The listing builds one solid part. Answer for the finished solid, in the listing's coordinates (mm). A direction names the side the tool comes from. Round coordinates to 2 decimals unless told otherwise and drop trailing zeros. Order: outer loops, then holes, each group sorted by start corner. A loop starts at its lowest first (then second) coordinate and runs counter-clockwise, first axis right, second up. Notation, with made-up numbers: (-18, 43) - (-1, 43) arc R25 ccw to (-1, 79) - close; hole circle Ø8 at (81.5, 70.25). An arc over 180 degrees is marked (long way). Write item = value, one per line.
from build123d import *

# Parameters (mm, degrees)
SKETCH1_W            = 20
SKETCH1_H            = 20
BOSS_EXTRUDE1_DEPTH  = 7.5
SKETCH1_3_W          = 20
SKETCH1_3_H          = 20
CUT_EXTRUDE2_DEPTH   = 1.5
SKETCH3_W            = 10
SKETCH3_H            = 20
BOSS_EXTRUDE2_DEPTH  = 1.5
SKETCH4_R            = 1.5
CUT_EXTRUDE3_DEPTH   = 5
MOUNTHOLE_DEPTH      = 17.007810594
MOUNTHOLE_DEPTH_BACK = 17.007810594
SKETCH5_R            = 1.5
SKETCH6_R            = 3
CUT_EXTRUDE5_DEPTH   = 1.25


with BuildPart() as part:
    # Sketch1 → Boss-Extrude1 (new, symmetric)
    with BuildSketch(Plane(origin=(0, 0, 0), x_dir=(1, 0, 0), z_dir=(0, 1, 0))):
        Rectangle(SKETCH1_W, SKETCH1_H)
    extrude(amount=BOSS_EXTRUDE1_DEPTH, both=True)

    # Sketch1_3 → Cut-Extrude2 (cut, symmetric)
    with BuildSketch(Plane(origin=(0, 0, 0), x_dir=(1, 0, 0), z_dir=(0, 1, 0))):
        Rectangle(SKETCH1_3_W, SKETCH1_3_H)
    extrude(amount=CUT_EXTRUDE2_DEPTH, both=True, mode=Mode.SUBTRACT)


with BuildPart() as cut_extrude2_piece_1:
    # of the separate pieces the step leaves, piece 1, a body of its own (cut_extrude2_pieces)
    add(part.part.solids().sort_by_distance((-10, -7.5, -10))[0])



with BuildPart() as cut_extrude2_piece_2:
    # of the separate pieces the step leaves, piece 2, a body of its own (cut_extrude2_pieces)
    add(part.part.solids().sort_by_distance((-10, 1.5, -10))[0])


with BuildPart() as cut_extrude2_piece_1_1:
    add(cut_extrude2_piece_1.part)

    add(cut_extrude2_piece_2.part)  # Boss-Extrude2 merges Cut-Extrude2 piece 2
    # Sketch3 → Boss-Extrude2 (add, symmetric)
    with BuildSketch(Plane(origin=(0, 0, 0), x_dir=(1, 0, 0), z_dir=(0, 1, 0))):
        with Locations((5, 0)):
            Rectangle(SKETCH3_W, SKETCH3_H)
    extrude(amount=BOSS_EXTRUDE2_DEPTH, both=True)

    # Sketch4 → Cut-Extrude3 (cut)
    with BuildSketch(Plane(origin=(10, 0, 0), x_dir=(0, 0, -1), z_dir=(1, 0, 0))):
        Circle(SKETCH4_R)
    extrude(amount=-CUT_EXTRUDE3_DEPTH, mode=Mode.SUBTRACT)

    # Sketch5 → mounthole (cut, two sides: drawn at the far end of the back side and taken through both)
    with BuildSketch(Plane(origin=(0, 0, 0), x_dir=(1, 0, 0), z_dir=(0, 1, 0)).offset(-MOUNTHOLE_DEPTH_BACK)):
        with Locations(Location((-5, 5, 0), (0, 0, 270))):
            Circle(SKETCH5_R)
        with Locations(Location((5, 5, 0), (0, 0, 270))):
            Circle(SKETCH5_R)
        with Locations(Location((5, -5, 0), (0, 0, 270))):
            Circle(SKETCH5_R)
        with Locations(Location((-5, -5, 0), (0, 0, 270))):
            Circle(SKETCH5_R)
    extrude(amount=MOUNTHOLE_DEPTH + MOUNTHOLE_DEPTH_BACK, mode=Mode.SUBTRACT)

    # Sketch6 → Cut-Extrude5 (cut, symmetric)
    with BuildSketch(Plane(origin=(5, 0, 0), x_dir=(0, 0, -1), z_dir=(1, 0, 0))):
        Circle(SKETCH6_R)
    extrude(amount=CUT_EXTRUDE5_DEPTH, both=True, mode=Mode.SUBTRACT)


solid = cut_extrude2_piece_1_1.part
Q1. Determine the mould class of faces 4 (the face through (-5, 1.5, 0)), 5 (the face through (-3.99, -4.54, -6.11)), 6 (the face through (0, -7.5, 0)) for opening direction Y: released by +Y, released by -Y, zero draft, split by the parting line, or undercut.
Model answer:
face_4 = undercut
face_5 = zero draft
face_6 = released by -Y
Q2. Section A-A on x = -2.75 is taken. Determine the outline of the cut face in (y, z).
Model answer:
outline = (-7.5, -10) - (-1.5, -10) - (-1.5, 10) - (-7.5, 10) - close; (1.5, -10) - (7.5, -10) - (7.5, 10) - (1.5, 10) - close
Q3. Section D-D on z = 5 is taken. Determine the outline of the cut face in (x, y), then the cut area to 3 significant figures.
Model answer:
outline = (-10, -7.5) - (-6.5, -7.5) - (-6.5, -1.5) - (-10, -1.5) - close; (-10, 1.5) - (-6.5, 1.5) - (-6.5, 7.5) - (-10, 7.5) - close; (-3.5, -7.5) - (3.5, -7.5) - (3.5, 7.5) - (-3.5, 7.5) - (-3.5, 1.5) - (0, 1.5) - (0, -1.5) - (-3.5, -1.5) - close; (6.5, -7.5) - (10, -7.5) - (10, 7.5) - (6.5, 7.5) - close
area = 189 mm^2
Q4. Section B-B on y = -5.5 is taken. Determine the outline of the cut face in (x, z), then the cut area to 3 significant figures.
Model answer:
outline = (-10, -10) - (10, -10) - (10, 10) - (-10, 10) - close; hole circle Ø3 at (-5, -5); hole circle Ø3 at (-5, 5); hole circle Ø3 at (5, -5); hole circle Ø3 at (5, 5)
area = 372 mm^2
Q5. Find the intervals of material crossed by line 1 (X direction, y = 3, z = -5); line 2 (Y direction, x = -8.75, z = 4); line 3 (X direction, y = -3.25, z = -5.75), in increasing order. Write a range as from..to.
Model answer:
line_1 = -10..-6.5, -3.5..3.5, 6.5..10
line_2 = -7.5..-1.5, 1.5..7.5
line_3 = -10..-6.3, -3.7..3.7, 6.3..10
Q6. Section C-C on x = -5 is taken. Determine the outline of the cut face in (y, z), then the cut area to 3 significant figures.
Model answer:
outline = (-7.5, -10) - (-1.5, -10) - (-1.5, -6.5) - (-7.5, -6.5) - close; (-7.5, -3.5) - (-1.5, -3.5) - (-1.5, 3.5) - (-7.5, 3.5) - close; (-7.5, 6.5) - (-1.5, 6.5) - (-1.5, 10) - (-7.5, 10) - close; (1.5, -10) - (7.5, -10) - (7.5, -6.5) - (1.5, -6.5) - close; (1.5, -3.5) - (7.5, -3.5) - (7.5, 3.5) - (1.5, 3.5) - close; (1.5, 6.5) - (7.5, 6.5) - (7.5, 10) - (1.5, 10) - close
area = 168 mm^2
Q7. Flat-ended cylindrical pins translate along their axes: P1, Ø1.5, axis at y = -0.5, z = -2, coming from the -X side; P2, Ø1.8, axis at x = -5, z = 5, coming from the -Y side. Find the tip coordinate at first contact, or state that the pin passes through.
Model answer:
P1 = 0
P2 = through
Q8. For faces 1 (the face through (6.25, -1.3, -1.3)), 2 (the face through (0, 2, -10)), 3 (the face through (0, 0, 0)), determine the directions among +Z, -Z, +X, -X, +Y, -Y from which every point of the face is accessible in a straight line to the end or side of a thin tool.
Model answer:
face_1 = none
face_2 = -Z, +X, -X, +Y, -Y
face_3 = +Z, -Z, -X
